from build123d import *

# Parameters (mm, degrees)
CROQUIS1_W              = 25
CROQUIS1_H              = 80
SALIENTE_EXTRUIR1_DEPTH = 3
CROQUIS2_W              = 4
CROQUIS2_H              = 80
SALIENTE_EXTRUIR2_DEPTH = 50
CHAFL_N1_SIZE           = 10
REDONDEO1_R             = 10
CROQUIS3_R              = 1.6
CROQUIS3_R_2            = 11
CORTAR_EXTRUIR1_DEPTH   = 50
CHAFL_N2_SIZE           = 3


with BuildPart() as part:
    # Croquis1 → Saliente-Extruir1 (new body)
    with BuildSketch(Plane.XY):
        Rectangle(CROQUIS1_W, CROQUIS1_H)
    extrude(amount=SALIENTE_EXTRUIR1_DEPTH)

    # Croquis2 → Saliente-Extruir2 (add)
    with BuildSketch(Plane.XY.offset(3)):
        with Locations((-10.5, 0)):
            Rectangle(CROQUIS2_W, CROQUIS2_H)
    extrude(amount=SALIENTE_EXTRUIR2_DEPTH)

    # Chaflán1
    chafl_n1_edges = [part.edges().sort_by_distance(p)[0] for p in [
        (-10.5, -40, 53),
        (-10.5, 40, 53),
    ]]
    chamfer(chafl_n1_edges, length=CHAFL_N1_SIZE)

    # Redondeo1
    redondeo1_edges = [part.edges().sort_by_distance(p)[0] for p in [
        (-10.5, 30, 53),
        (-10.5, -30, 53),
        (-10.5, -40, 43),
        (-10.5, 40, 43),
    ]]
    fillet(redondeo1_edges, radius=REDONDEO1_R)

    # Croquis3 → Cortar-Extruir1 (cut)
    with BuildSketch(Plane.ZY.offset(12.5)):
        with Locations((11, 15.5)):
            Circle(CROQUIS3_R)
        with Locations((42, 15.5)):
            Circle(CROQUIS3_R)
        with Locations((11, -15.5)):
            Circle(CROQUIS3_R)
        with Locations((42, -15.5)):
            Circle(CROQUIS3_R)
        with Locations((26.5, 0)):
            Circle(CROQUIS3_R_2)
    extrude(amount=-CORTAR_EXTRUIR1_DEPTH, mode=Mode.SUBTRACT)

    # Chaflán2
    chafl_n2_edges = [part.edges().sort_by_distance(p)[0] for p in [
        (-12.5, 0, 15.5),
    ]]
    chamfer(chafl_n2_edges, length=CHAFL_N2_SIZE)


solid = part.part
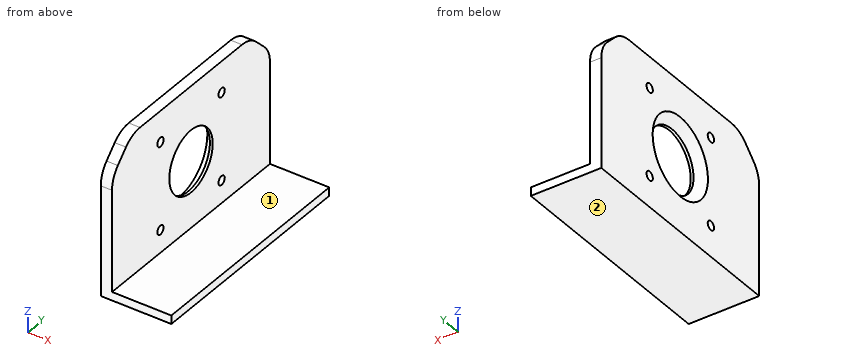
For this review, take the finished solid that the model builds, in its own axes (mm). Face numbers are marked on the shaded views. A direction names the side the tool comes from. Give positions to 0.01 mm unless a question says otherwise; leave off trailing zeros. Loops run counter-clockwise (first coordinate to the right, second up) from the corner with the lowest first, then second, coordinate; pieces in that order, holes last. Notation, with made-up numbers: M -34.75,80 L 15.25,80 A25 cw 15.25,113 Z; hole C 39.5,59.25 d5. An arc over 180 degrees is marked long. Answer as a JSON object with one key per item and string values. Group by question number.
Q1. For probe 1 along Y at (x, z) = (-10.1, 11); probe 2 along Z at (x, y) = (-2.5, 35); probe 3 along X at (y, z) = (-24.5, 8), list the stretches that pass through material, from the lowest coordinate up. Write a range as [from, to].
Q2. Add section A-A on z = 11. Give the boundary of the cut face in (x, y).
Q3. Add section B-B on y = 0. Give the boundary of the cut face in (x, z).
Q4. Tool access review of the marked faces 1 and 2: name each direction out of +Z, -Z, +X, -X, +Y, -Y from which nothing blocks a thin tool from reaching the whole face with its end or side.
Q5. Insertion check: P1, Ø10, axis at x = 6.5, y = -31.5, coming from the +Z side; P2, Ø2, axis at y = 25, z = 8.5, coming from the +X side. Each pin has a flat end and moves straight along its axis. Give the tip position at first contact, or say it passes through.
Q6. Add section C-C on z = 26.5. Give the boundary of the cut face in (x, y).
Q7. Add section D-D on y = -15.5. Give the boundary of the cut face in (x, z).
Checked values:
{
 "1": {"probe 1": "[-40, -17.1], [-13.9, 13.9], [17.1, 40]", "probe 2": "[0, 3]", "probe 3": "[-12.5, -8.5]"},
 "2": {"outline": "M -12.5,-40 L -8.5,-40 L -8.5,-17.1 L -12.5,-17.1 Z; M -12.5,-13.9 L -8.5,-13.9 L -8.5,13.9 L -12.5,13.9 Z; M -12.5,17.1 L -8.5,17.1 L -8.5,40 L -12.5,40 Z"},
 "3": {"outline": "M -12.5,0 L 12.5,0 L 12.5,3 L -8.5,3 L -8.5,15.5 L -9.5,15.5 L -12.5,12.5 Z; M -12.5,40.5 L -9.5,37.5 L -8.5,37.5 L -8.5,53 L -12.5,53 Z"},
 "4": {"face 1": "+Z, +X, +Y, -Y", "face 2": "-Z, +X, -X, +Y, -Y"},
 "5": {"P1": "z = 3", "P2": "x = -8.5"},
 "6": {"outline": "M -12.5,-40 L -8.5,-40 L -8.5,-11 L -9.5,-11 L -12.5,-14 Z; M -12.5,14 L -9.5,11 L -8.5,11 L -8.5,40 L -12.5,40 Z"},
 "7": {"outline": "M -12.5,0 L 12.5,0 L 12.5,3 L -8.5,3 L -8.5,9.4 L -12.5,9.4 Z; M -12.5,12.6 L -8.5,12.6 L -8.5,40.4 L -12.5,40.4 Z; M -12.5,43.6 L -8.5,43.6 L -8.5,53 L -12.5,53 Z"}
}
